Source: CAD feature listing. Evaluate the final solid. Frame: model axes, mm. Give positions to 0.01 mm unless a question says otherwise; leave off trailing zeros. Order: outer loops, then holes, each group sorted by start corner. A loop starts at its lowest first (then second) coordinate and runs counter-clockwise, first axis right, second up.
1) Section C-C, the plane x = 110. Return loops of the section in (y, z), plus the area to 3 significant figures.
2) Section A-A, the plane x = 48. Return loops of the section in (y, z).
3) First-contact query: P1, Ø1, axis at y = -90, z = 1.5, coming from the +X side; P2, Ø10.5, axis at x = 307.12, y = -83.9, coming from the -Z side; P3, Ø2, axis at y = -83, z = 2.5, coming from the -X side. Flat tips, straight axial feed; report the tip coordinate or a pass-through.
4) Draft query along Y for faces 1 (the face through (301.116, -81.409, 2.348)), 2 (the face through (174, -75, 4.762)), 3 (the face through (372.01, -83.72, 2.41)), 4 (the face through (117.158, -79.944, 2.348)). Return one class per face: released by +Y, released by -Y, zero draft, split by the parting line, or undercut.
5) Material intervals for line 1 (Y direction, x = 240, z = 3.15); line 2 (Y direction, x = 45, z = 3.5); line 3 (X direction, y = -76.5, z = 2.6), sorted ascending.
6) Section B-B, the plane z = 2.6. Return loops of the section in (x, y), plus the area to 3 significant figures.
```python
from build123d import *

# Parameters (mm, degrees)
BOSS_EXTRUDE1_DEPTH = 4.7625
SKETCH1_4_R         = 6.5
CUT_EXTRUDE1_DEPTH  = 439.920211962
CUT_EXTRUDE5_DEPTH  = 10
FILLET1_R           = 48
CUT_EXTRUDE6_DEPTH  = 10


with BuildPart() as part:
    # Sketch1 → Boss-Extrude1 (new body)
    with BuildSketch(Plane.XY):
        Polygon((428.120588235, 28.570833333), (0, 28.570833333), (-98.879411765, 3.850980392), (-31.879411765, -96.649019608), (366, -96.649019608), (403.120588235, -71.149019608), align=None)
    extrude(amount=BOSS_EXTRUDE1_DEPTH)

    # Sketch1_4 → Cut-Extrude1 (cut, through all)
    with BuildSketch(Plane.XY):
        with Locations(Location((-16, -83.899019608, 0), (0, 0, 180))):
            Circle(SKETCH1_4_R)
        with Locations(Location((48, -83.899019608, 0), (0, 0, 180))):
            Circle(SKETCH1_4_R)
        with Locations(Location((112, -83.899019608, 0), (0, 0, 180))):
            Circle(SKETCH1_4_R)
        with Locations(Location((176, -83.899019608, 0), (0, 0, 180))):
            Circle(SKETCH1_4_R)
        with Locations(Location((240, -83.899019608, 0), (0, 0, 180))):
            Circle(SKETCH1_4_R)
        with Locations(Location((307.120588235, -83.899019608, 0), (0, 0, 180))):
            Circle(SKETCH1_4_R)
    extrude(amount=CUT_EXTRUDE1_DEPTH, mode=Mode.SUBTRACT)

    # Sketch8 → Cut-Extrude5 (cut)
    with BuildSketch(Plane.XY.offset(4.7625)):
        Polygon((-48.879411765, -71.149019608), (403.120588235, -71.149019608), (428.120588235, 28.570833333), (0, 28.570833333), (-98.879411765, 3.850980392), align=None)
    extrude(amount=-CUT_EXTRUDE5_DEPTH, mode=Mode.SUBTRACT)

    # Fillet1
    fillet1_edges = [part.edges().sort_by_distance(p)[0] for p in [
        (-31.879411765, -96.649019608, 2.38125),
    ]]
    fillet(fillet1_edges, radius=FILLET1_R)

    # Sketch9 → Cut-Extrude6 (cut)
    with BuildSketch(Plane.XY.offset(4.7625)):
        Polygon((403.120588235, -71.149019608), (340.005873473, -96.649019608), (366, -96.649019608), align=None)
    extrude(amount=-CUT_EXTRUDE6_DEPTH, mode=Mode.SUBTRACT)


solid = part.part
```
From the geometry:
1. outline: (-96.65, 0) - (-90.08, 0) - (-90.08, 4.76) - (-96.65, 4.76) - close; (-77.71, 0) - (-71.15, 0) - (-71.15, 4.76) - (-77.71, 4.76) - close
1. area: 62.5 mm2
2. outline: (-96.65, 0) - (-90.4, 0) - (-90.4, 4.76) - (-96.65, 4.76) - close; (-77.4, 0) - (-71.15, 0) - (-71.15, 4.76) - (-77.4, 4.76) - close
3. P1: stops at x = 357.7
3. P2: passes through
3. P3: stops at x = -40.71
4. face 1: undercut
4. face 2: zero draft
4. face 3: released by -Y
4. face 4: undercut
5. line 1: y = -96.65 to -90.4, -77.4 to -71.15
5. line 2: y = -96.65 to -89.67, -78.13 to -71.15
5. line 3: x = -45.28 to 389.88
6. outline: (-48.88, -71.15) - (-46.13, -75.27) arc R48 ccw to (-6.19, -96.65) - (340.01, -96.65) - (403.12, -71.15) - close; hole circle Ø13 at (-16, -83.9); hole circle Ø13 at (48, -83.9); hole circle Ø13 at (112, -83.9); hole circle Ø13 at (176, -83.9); hole circle Ø13 at (240, -83.9); hole circle Ø13 at (307.12, -83.9)
6. area: 9,610 mm2
